from build123d import *

# Parameters (mm, degrees)
MODEL_R             = 1.5
MODEL_W             = 6
MODEL_H             = 2
BOSS_EXTRUDE1_DEPTH = 2
SKETCH15_W          = 2
SKETCH15_H          = 3
CUT_EXTRUDE1_DEPTH  = 2


with BuildPart() as part:
    # Model → Boss-Extrude1 (new body)
    with BuildSketch(Plane.XY):
        with BuildLine():
            Line((6.363961031, 1.171572875), (2.828427125, 4.707106781))
            Line((2.828427125, 4.707106781), (0, 1.878679656))
            Line((0, 1.878679656), (0, -1.878679656))
            ThreePointArc((0, -1.878679656), (0.878679656, -4), (3, -4.878679656))
            Line((3, -4.878679656), (5.828427125, -4.878679656))
            Line((5.828427125, -4.878679656), (6.156854249, -4.878679656))
            ThreePointArc((6.156854249, -4.878679656), (8.278174593, -5.757359313), (9.156854249, -7.878679656))
            Line((9.156854249, -7.878679656), (9.156854249, -8.641362585))
            ThreePointArc((9.156854249, -8.641362585), (10.035533906, -10.762682929), (12.156854249, -11.641362585))
            Line((12.156854249, -11.641362585), (21.156854249, -11.641362585))
            ThreePointArc((21.156854249, -11.641362585), (23.985281374, -10.46978971), (25.156854249, -7.641362585))
            Line((25.156854249, -7.641362585), (25.156854249, 8.949747468))
            Line((25.156854249, 8.949747468), (14.01040764, 8.949747468))
            Line((14.01040764, 8.949747468), (14.01040764, 12.949747468))
            Line((14.01040764, 12.949747468), (7.071067812, 12.949747468))
            Line((7.071067812, 12.949747468), (7.071067812, 8.949747468))
            Line((7.071067812, 8.949747468), (8.485281374, 7.535533906))
            Line((8.485281374, 7.535533906), (5.656854249, 4.707106781))
            Line((5.656854249, 4.707106781), (7.778174593, 2.585786438))
            Line((7.778174593, 2.585786438), (6.363961031, 1.171572875))
        make_face()
        with Locations((16.191687414, -5.558946351)):
            Circle(MODEL_R, mode=Mode.SUBTRACT)
        with Locations((18.156854249, 5.949747468)):
            Rectangle(MODEL_W, MODEL_H, mode=Mode.SUBTRACT)
    extrude(amount=BOSS_EXTRUDE1_DEPTH)

    # Sketch15 → Cut-Extrude1 (cut)
    with BuildSketch(Plane(origin=(5.181980515, 5.181980515, 0), x_dir=(0, 0, 1), z_dir=(-0.707106781, -0.707106781, 0))):
        with Locations((1, -2.171572875)):
            Rectangle(SKETCH15_W, SKETCH15_H)
    extrude(amount=-CUT_EXTRUDE1_DEPTH, mode=Mode.SUBTRACT)


solid = part.part
Verification items for the finished model (mm, model axes). A direction names the side the tool comes from. Round coordinates to 2 decimals unless told otherwise and drop trailing zeros. Write each loop counter-clockwise with the first axis right and the second up, starting at its lowest first coordinate (ties: lowest second). Pieces come first, ordered by that corner, then holes.
(1) Mould release check, pull along Y, two halves, no side actions. Record for faces 4 (the flat face through (25.157, 1, 1)), 5 (the cylindrical face through (8.25, -5.73, 0.99)), 6 (the flat face through (18, 6.95, 1)): pulls with the +Y half, pulls with the -Y half, needs draft (parallel to the pull), parting line crosses it, or undercut.
Returned:
face 4: needs draft
face 5: pulls with the -Y half
face 6: undercut
(2) Section check A-A (x = 19). Enter the section's corners in (y, z).
Returned:
outline: (-11.64, 0) - (4.95, 0) - (4.95, 2) - (-11.64, 2) - close; (6.95, 0) - (8.95, 0) - (8.95, 2) - (6.95, 2) - close
(3) Section check D-D (z = 1.1). Enter the section's corners in (x, y), plus the area to 3 significant figures.
Returned:
outline: (0, -1.88) arc R3 ccw to (3, -4.88) - (6.16, -4.88) arc R3 cw to (9.16, -7.88) - (9.16, -8.64) arc R3 ccw to (12.16, -11.64) - (21.16, -11.64) arc R4 ccw to (25.16, -7.64) - (25.16, 8.95) - (14.01, 8.95) - (14.01, 12.95) - (7.07, 12.95) - (7.07, 8.95) - (8.49, 7.54) - (7.07, 6.12) - (9.19, 4) - (6.36, 1.17) - (2.83, 4.71) - (0, 1.88) - close; hole circle Ø3 at (16.19, -5.56); hole (15.16, 4.95) - (21.16, 4.95) - (21.16, 6.95) - (15.16, 6.95) - close
area: 410 mm2
(4) Material ranges on line 1 (Y direction, x = 19.25, z = 1.7); line 2 (Y direction, x = 17.5, z = 1.55); line 3 (X direction, y = -6.25, z = 1.4), recorded low to high.
Returned:
line 1: y = -11.64 to 4.95, 6.95 to 8.95
line 2: y = -11.64 to -6.29, -4.83 to 4.95, 6.95 to 8.95
line 3: x = 8.68 to 14.86, 17.52 to 25.16
(5) Access from +Z, -Z, +X, -X, +Y, -Y to the whole of each face (thin tool, end or side, straight path). Record for faces 1 (the flat face through (18, 4.95, 1)), 2 (the flat face through (20, 8.95, 1)), 3 (the flat face through (7.79, 6.84, 0.99)).
Returned:
face 1: +Z, -Z
face 2: +Z, -Z, +X, +Y
face 3: +Z, -Z, -X
(6) Depth check by flat-ended pin: pin 1 Ø0.6 at (y, z) = (6.5, 1) entering from -X; pin 2 Ø0.6 at (y, z) = (-8.5, 0.5) entering from -X; pin 3 Ø0.6 at (x, z) = (19.5, 1.5) entering from +Y. Enter the tip coordinate at first touch or a pass-through.
Returned:
pin 1: stops at x = 7.15
pin 2: stops at x = 9.16
pin 3: stops at y = 8.95
(7) Section check C-C (x = 16.25). Enter the section's corners in (y, z), plus the area to 3 significant figures.
Returned:
outline: (-11.64, 0) - (-7.06, 0) - (-7.06, 2) - (-11.64, 2) - close; (-4.06, 0) - (4.95, 0) - (4.95, 2) - (-4.06, 2) - close; (6.95, 0) - (8.95, 0) - (8.95, 2) - (6.95, 2) - close
area: 31.2 mm2
(8) Section check B-B (y = 3). Enter the section's corners in (x, z).
Returned:
outline: (1.12, 0) - (4.54, 0) - (4.54, 2) - (1.12, 2) - close; (8.19, 0) - (25.16, 0) - (25.16, 2) - (8.19, 2) - close
